Here's how the part is built. I have some questions about the finished solid (model axes, mm). A direction names the side the tool comes from. Round coordinates to 2 decimals unless told otherwise and drop trailing zeros. Order: outer loops, then holes, each group sorted by start corner. A loop starts at its lowest first (then second) coordinate and runs counter-clockwise, first axis right, second up. Notation, with made-up numbers: (48, 40) -> (94, 40) arc R26 ccw to (94, 69) -> close; hole circle Ø8 at (-29.5, -8). An arc over 180 degrees is marked (long way). Answer in a Markdown table with one row per item.
```python
from build123d import *

# Parameters (mm, degrees)
ESQUISSE1_R        = 41.275
BOSS_EXTRU_1_DEPTH = 158.75
CONG_1_R           = 10


with BuildPart() as part:
    # Esquisse1 → Boss.-Extru.1 (new body)
    with BuildSketch(Plane(origin=(0, 0, 0), x_dir=(1, 0, 0), z_dir=(0, 1, 0))):
        with Locations(Location((0, 0, 0), (0, 0, 90))):
            Circle(ESQUISSE1_R)
    extrude(amount=BOSS_EXTRU_1_DEPTH)

    # Esquisse2 → Révolution1 (revolve)
    with BuildSketch(Plane.XY, mode=Mode.PRIVATE) as r_volution1_sk:
        with BuildLine():
            Line((18.489381751, 188.598064752), (30.542749869, 179.829366122))
            ThreePointArc((30.542749869, 179.829366122), (38.437502567, 170.577096738), (41.275, 158.75))
            Line((41.275, 158.75), (0, 158.75))
            Line((0, 158.75), (0, 247.65))
            Line((0, 247.65), (15.875, 247.65))
            Line((15.875, 247.65), (15.875, 193.733009377))
            ThreePointArc((15.875, 193.733009377), (16.56621586, 190.851922419), (18.489381751, 188.598064752))
        make_face()
    revolve(r_volution1_sk.sketch.rotate(Axis((0, 247.65, 0), (0, -1, 0)), 180), axis=Axis((0, 247.65, 0), (0, -1, 0)))

    # Congé1
    cong_1_edges = [part.edges().sort_by_distance(p)[0] for p in [
        (0, 0, 41.275),
    ]]
    fillet(cong_1_edges, radius=CONG_1_R)


solid = part.part
```
1. Please list where these lines run through material, in increasing order: line 1 along X through (y, z) = (155.5, 34.5); line 2 along Y through (x, z) = (29.5, 9); line 3 along X through (y, z) = (107, -35).
Numbers:
| item | result |
|---|---|
| line 1 | x = -22.66 to 22.66 |
| line 2 | y = 0 to 179.61 |
| line 3 | x = -21.88 to 21.88 |
2. For faces 1 (the face through (0, 247.65, 0)), 2 (the face through (3.441, 220.314, 15.497)), which set-ups out of +Z, -Z, +X, -X, +Y, -Y let a thin tool reach every point of the face, with its end or its side?
Numbers:
| item | result |
|---|---|
| face 1 | +Z, -Z, +X, -X, +Y |
| face 2 | +Y |
3. For pin 1 Ø2 at (x, y) = (-8, 203.5) entering from +Z; pin 2 Ø4 at (y, z) = (185, -13) entering from -X; pin 3 Ø4 at (y, z) = (30, -22) entering from -X, each with a flat end and sliding along its axis, tell me the tip position at first contact or that it passes through.
Numbers:
| item | result |
|---|---|
| pin 1 | stops at z = 14.25 |
| pin 2 | stops at x = -22.92 |
| pin 3 | stops at x = -36.11 |
4. Suppose I cut it at A-A on y = 145.5. Write out the boundary of the cut face in (x, z) (3 decimals), then the cut area to 3 significant figures.
Numbers:
| item | result |
|---|---|
| outline | circle Ø82.55 at (0, 0) |
| area | 5,350 mm2 |
